```python
from build123d import *

# Parameters (mm, degrees)
F0_W     = 410
F0_H     = 110
F1_DEPTH = 7
F2_W     = 45
F2_H     = 45
F3_DEPTH = 25
F0_W_2   = 15
F4_DEPTH = 7


# Not quite as in the source:
# - a feature names something its author has since deleted; it is built from what else it names


with BuildPart() as f1:
    # F0 (on Top) → F1 (new body)
    with BuildSketch(Plane.XY):
        Rectangle(F0_W, F0_H)
    extrude(amount=F1_DEPTH)

    # F2 (on face) → F3 (cut)
    with BuildSketch(Plane.XY.offset(7)):
        with Locations((-60, 0)):
            Rectangle(F2_W, F2_H)
        with Locations((45, 0)):
            Rectangle(F2_W, F2_H)
        with Locations((150, 0)):
            Rectangle(F2_W, F2_H)
        with Locations((-165, 0)):
            Rectangle(F2_W, F2_H)
    extrude(amount=-F3_DEPTH, mode=Mode.SUBTRACT)

    # F0 (on Top) → F4 (join)
    with BuildSketch(Plane.XY):
        with Locations((-212.5, 0)):
            Rectangle(F0_W_2, F0_H)
    extrude(amount=F4_DEPTH)


solid = f1.part
```
Design review of the part built by this model. Coordinates are the model's own, in mm. A direction names the side the tool comes from. Coordinates: 2 decimals unless noted, no trailing zeros. Write each loop counter-clockwise with the first axis right and the second up, starting at its lowest first coordinate (ties: lowest second). Pieces come first, ordered by that corner, then holes.
1) Add section A-A (x = 143.5). Write out the cut boundary in (y, z).
2) Machinability: for faces 1 (the flat face through (-220, -1, 3)), 2 (the flat face through (-60, -22.5, 4)), which of the approach directions +Z, -Z, +X, -X, +Y, -Y give a long, thin tool a straight path to every point of the face, cutting with its end or side? Answer none if there is none.
3) Add section C-C (z = 5.75). Write out the cut boundary in (x, y), plus the area to 4 significant figures.
4) Mouldability with a two-part tool opening along Y and no side actions: class faces 3 (the flat face through (-10, -55, 3)), 4 (the flat face through (-10, 1, 7)), 5 (the flat face through (150, -22.5, 4)), 6 (the flat face through (-10, 55, 3)) as +Y half, -Y half, draft (parallel to the pull), parting line (faces both ways), or undercut.
5) Add section B-B (y = -11.5). Write out the cut boundary in (x, z).
6) To check wall thickness, follow L1, parallel to X at y = -22, z = 4; L2, parallel to Y at x = 169, z = 4.5. State the ranges of each line that lie inside material, in increasing order.
Check result:
1. outline: (-55, 0) - (-22.5, 0) - (-22.5, 7) - (-55, 7) - close; (22.5, 0) - (55, 0) - (55, 7) - (22.5, 7) - close
2. face 1: +Z, -Z, -X, +Y, -Y
2. face 2: +Z, -Z
3. outline: (-220, -55) - (205, -55) - (205, 55) - (-220, 55) - close; hole (-187.5, -22.5) - (-142.5, -22.5) - (-142.5, 22.5) - (-187.5, 22.5) - close; hole (-82.5, -22.5) - (-37.5, -22.5) - (-37.5, 22.5) - (-82.5, 22.5) - close; hole (22.5, -22.5) - (67.5, -22.5) - (67.5, 22.5) - (22.5, 22.5) - close; hole (127.5, -22.5) - (172.5, -22.5) - (172.5, 22.5) - (127.5, 22.5) - close
3. area: 38,650 mm2
4. face 3: -Y half
4. face 4: draft
4. face 5: undercut
4. face 6: +Y half
5. outline: (-220, 0) - (-187.5, 0) - (-187.5, 7) - (-220, 7) - close; (-142.5, 0) - (-82.5, 0) - (-82.5, 7) - (-142.5, 7) - close; (-37.5, 0) - (22.5, 0) - (22.5, 7) - (-37.5, 7) - close; (67.5, 0) - (127.5, 0) - (127.5, 7) - (67.5, 7) - close; (172.5, 0) - (205, 0) - (205, 7) - (172.5, 7) - close
6. L1: x = -220 to -187.5, -142.5 to -82.5, -37.5 to 22.5, 67.5 to 127.5, 172.5 to 205
6. L2: y = -55 to -22.5, 22.5 to 55
